Model file for the job. Use its own axes, mm. Coordinates: 2 decimals unless noted, no trailing zeros. Use CSV: the item, a comma, the result in double quotes. Start each with the question number.
(1) Probe L1, parallel to X at y = 121, z = 171; L2, parallel to Y at x = 49, z = 168.5; L3, parallel to Y at x = 57.5, z = 156. List the from-to ranges inside material, lowest first.
(2) Cut at A-A on x = 61.25. Give the number of separate pieces and of enclosed holes in the cut face, plus the area to 3 significant figures.
(3) Pull direction Z, two halves, no side cores. Call faces 1 (the cylindrical face through (63.44, 61.85, 126.89)), 2 (the cylindrical face through (57.73, 92.56, 158.14)): pulls with the +Z half, pulls with the -Z half, needs draft (parallel to the pull), parting line crosses it, or undercut.
(4) Pin check, flat tips, straight feed: pin 1 Ø1 at (x, z) = (58.5, 137.5) entering from -Y; pin 2 Ø5 at (x, y) = (49, 124) entering from +Z; pin 3 Ø3 at (x, z) = (56.5, 134) entering from +Y. Stop position of each tip, or through.
```python
from build123d import *

# Parameters (mm, degrees)
SKETCH1_R                = 5
SKETCH1_R_2              = 4
BOSS_EXTRUDE1_DEPTH      = 80
BOSS_EXTRUDE1_DEPTH_BACK = 30
SKETCH2_R                = 3
CUT_EXTRUDE1_DEPTH       = 58.904930039
CUT_EXTRUDE1_DEPTH_BACK  = 58.904930039


with BuildPart() as part:
    # Sketch1 → Boss-Extrude1 (new body, two sides)
    with BuildSketch(Plane(origin=(-18.263591419, 106.35230846, 73.959767463), x_dir=(0.989737493, 0.132142803, 0.054387259), z_dir=(-0.139606326, 0.812953742, 0.565346165))) as boss_extrude1_sk:
        with Locations((75.664084078, -74.988676697)):
            Circle(SKETCH1_R)
        with Locations((75.664084078, -74.988676697)):
            Circle(SKETCH1_R_2, mode=Mode.SUBTRACT)
    extrude(amount=BOSS_EXTRUDE1_DEPTH)
    extrude(boss_extrude1_sk.sketch, amount=-BOSS_EXTRUDE1_DEPTH_BACK)

    # Sketch2 → Cut-Extrude1 (cut, two sides)
    with BuildSketch(Plane(origin=(167.461192563, -27.829766449, 89.299122305), x_dir=(0.974445609, 0.011329449, 0.22433769), z_dir=(-0.175971104, -0.582218049, 0.793760867))) as cut_extrude1_sk:
        with Locations((-93.296905198, 111.340129179)):
            Circle(SKETCH2_R)
    extrude(amount=CUT_EXTRUDE1_DEPTH, mode=Mode.SUBTRACT)
    extrude(cut_extrude1_sk.sketch, amount=-CUT_EXTRUDE1_DEPTH_BACK, mode=Mode.SUBTRACT)


solid = part.part
```
Outcome:
1,L1,"46.07 to 47.12, 54.75 to 55.81"
1,L2,"108.86 to 111.04, 121.05 to 123.23"
1,L3,"88.84 to 90.92, 101.6 to 103.68"
2,separate pieces,"3"
2,enclosed holes,"0"
2,area,"117 mm2"
3,face 1,"undercut"
3,face 2,"parting line crosses it"
4,pin 1,"y = 61.7"
4,pin 2,"z = 182.51"
4,pin 3,"y = 75.53"
